The figure shows three views and two pictorial views of one solid part (mm, origin at its lowest corner). Answer the questions. Round coordinates to 2 decimals unless told otherwise and drop trailing zeros. Write each loop counter-clockwise with the first axis right and the second up, starting at its lowest first coordinate (ties: lowest second). Pieces come first, ordered by that corner, then holes. Notation, with made-up numbers: M 88,9 L 112,9 A17 cw 112,34 Z; hole C -3.5,16 d4. An arc over 180 degrees is marked long. Answer in a Markdown table with one row per item.
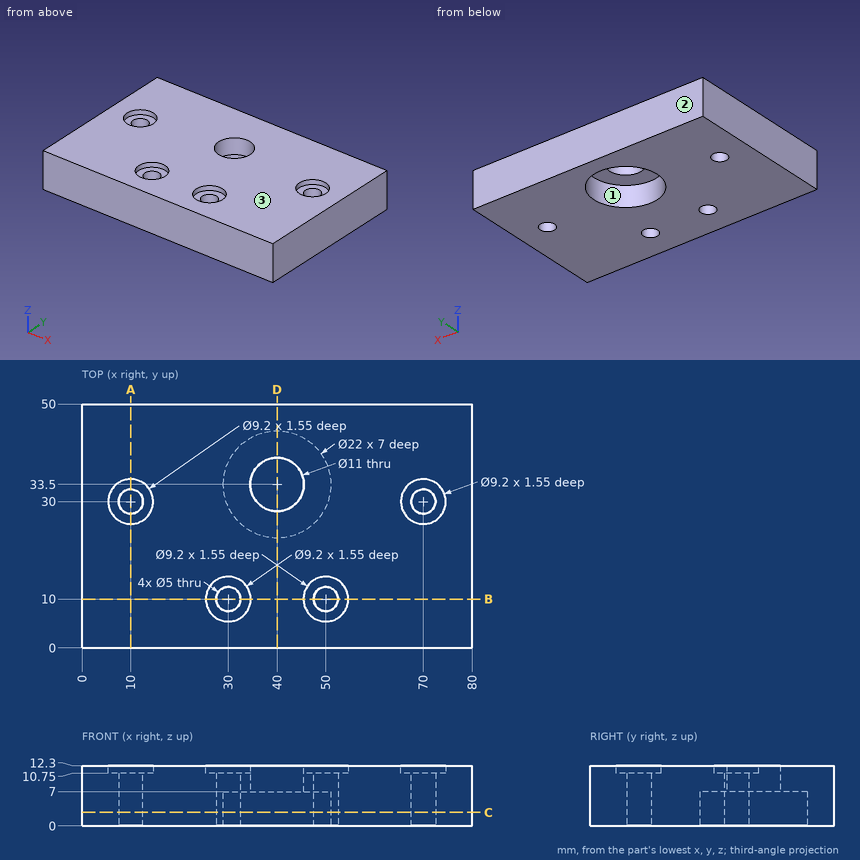
1. The part is cut by section A-A (x = 10). Determine the outline of the cut face in (y, z), plus the area to 3 significant figures.
Calculated:
| item | result |
|---|---|
| outline | M 0,0 L 27.5,0 L 27.5,10.75 L 25.4,10.75 L 25.4,12.3 L 0,12.3 Z; M 32.5,0 L 50,0 L 50,12.3 L 34.6,12.3 L 34.6,10.75 L 32.5,10.75 Z |
| area | 547 mm² |
2. Given pin 1 (5.5 mm diameter, centred on x = 30, y = 10, fed in from +Z); pin 2 (11 mm diameter, centred on x = 36, y = 36.5, fed in from -Z), each flat-ended and moving along its own axis, determine where each tip first touches the part or whether it passes through.
Calculated:
| item | result |
|---|---|
| pin 1 | stops at z = 10.75 |
| pin 2 | stops at z = 7 |
3. Consider line 1 along Y through (x, z) = (30, 11.15); line 2 along X through (y, z) = (31, 1); line 3 along X through (y, z) = (9, 9.5). Determine where each line is inside the solid, lowest interval first. Write a range as from..to.
Calculated:
| item | result |
|---|---|
| line 1 | y = 0..5.4, 14.6..50 |
| line 2 | x = 0..7.71, 12.29..29.29, 50.71..67.71, 72.29..80 |
| line 3 | x = 0..27.71, 32.29..47.71, 52.29..80 |
4. The part is cut by section B-B (y = 10). Determine the outline of the cut face in (x, z).
Calculated:
| item | result |
|---|---|
| outline | M 0,0 L 27.5,0 L 27.5,10.75 L 25.4,10.75 L 25.4,12.3 L 0,12.3 Z; M 32.5,0 L 47.5,0 L 47.5,10.75 L 45.4,10.75 L 45.4,12.3 L 34.6,12.3 L 34.6,10.75 L 32.5,10.75 Z; M 52.5,0 L 80,0 L 80,12.3 L 54.6,12.3 L 54.6,10.75 L 52.5,10.75 Z |
5. The part is cut by section D-D (x = 40). Determine the outline of the cut face in (y, z), plus the area to 3 significant figures.
Calculated:
| item | result |
|---|---|
| outline | M 0,0 L 22.5,0 L 22.5,7 L 28,7 L 28,12.3 L 0,12.3 Z; M 39,7 L 44.5,7 L 44.5,0 L 50,0 L 50,12.3 L 39,12.3 Z |
| area | 403 mm² |
6. The part is cut by section C-C (z = 2.75). Determine the outline of the cut face in (x, y).
Calculated:
| item | result |
|---|---|
| outline | M 0,0 L 80,0 L 80,50 L 0,50 Z; hole C 10,30 d5; hole C 30,10 d5; hole C 40,33.5 d22; hole C 50,10 d5; hole C 70,30 d5 |
7. Determine the mould class of the marked faces 1, 2 and 3 for opening direction Y: released by +Y, released by -Y, zero draft, split by the parting line, or undercut.
Calculated:
| item | result |
|---|---|
| face 1 | undercut |
| face 2 | released by +Y |
| face 3 | zero draft |
